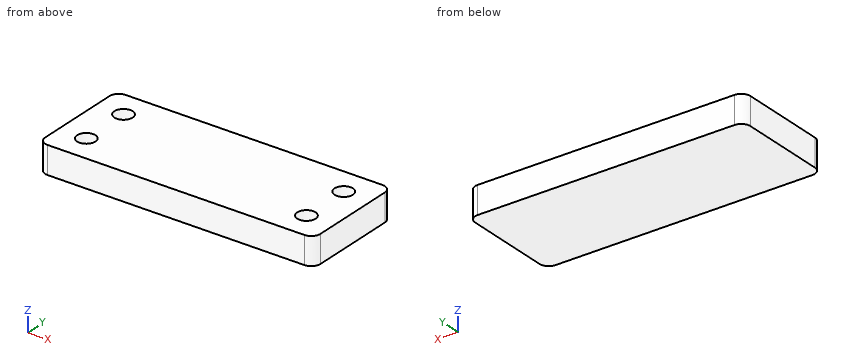
Solid Edge part; units mm, degrees
sketch "Sketch1" plane through (0, 0, 0) normal (0, 0, 1) x (1, 0, 0)
  line L0 (-15, 5.75) -> (15, 5.75)
  line L1 (15, 5.75) -> (15, -5.75)
  line L2 (15, -5.75) -> (-15, -5.75)
  line L3 (-15, -5.75) -> (-15, 5.75)
  dimension "D1" = 15
  dimension "D2" = 15
extrude "Protrusion1" add sketch "Sketch1" along normal blind 3
fillet "Avrundningar_1" radius 1 4 edges at (-15, -5.75, 1.5) (15, -5.75, 1.5) (15, 5.75, 1.5) (-15, 5.75, 1.5)
sketch "Sketch2" plane through (0, 0, 3) normal (0, 0, 1) x (0, 1, 0)
  circle A0 centre (-2.75, 12) radius 1
  circle A1 centre (2.75, 12) radius 1
  circle A2 centre (2.75, -12) radius 1
  circle A3 centre (-2.75, -12) radius 1
  dimension "D1" = 2.75
  dimension "D2" = 2.75
extrude "Utskärning_fäste_fjädrar" cut sketch "Sketch2" against normal blind 1.5
Here's how the part is built. I have some questions about the finished solid (model axes, mm). Round coordinates to 2 decimals unless told otherwise and drop trailing zeros. Order: outer loops, then holes, each group sorted by start corner. A loop starts at its lowest first (then second) coordinate and runs counter-clockwise, first axis right, second up. Notation, with made-up numbers: M -26.5,-35.5 L -22.5,-35.5 A18 cw -22.5,-4.5 Z; hole C 51.5,-33.5 d11. An arc over 180 degrees is marked long. One line per question, with ' | ' between items.
1) Imagine slicing it at B-B, the plane x = -12. Write out the boundary of the cut face in (y, z), plus the area to 3 significant figures.
Checked values:
outline: M -5.75,0 L 5.75,0 L 5.75,3 L 3.75,3 L 3.75,1.5 L 1.75,1.5 L 1.75,3 L -1.75,3 L -1.75,1.5 L -3.75,1.5 L -3.75,3 L -5.75,3 Z | area: 28.5 mm²
2) Imagine slicing it at C-C, the plane y = 2.75. Write out the boundary of the cut face in (x, z), plus the area to 3 significant figures.
Checked values:
outline: M -15,0 L 15,0 L 15,3 L 13,3 L 13,1.5 L 11,1.5 L 11,3 L -11,3 L -11,1.5 L -13,1.5 L -13,3 L -15,3 Z | area: 84.0 mm²
3) I need wall thicknesses on line 1 (Y direction, x = 12, z = 2.6); line 2 (X direction, y = -2.75, z = 1.9); line 3 (X direction, y = 5.25, z = 0.3). Which ranges of each line are inside material? Lowest first, please.
Checked values:
line 1: y = -5.75 to -3.75, -1.75 to 1.75, 3.75 to 5.75 | line 2: x = -15 to -13, -11 to 11, 13 to 15 | line 3: x = -14.87 to 14.87
4) I'm going to push a flat-ended pin straight in: pin 1 Ø0.6 at (x, y) = (12, -2.5) entering from +Z. Where does the tip first touch, or does it pass through?
Checked values:
pin 1: stops at z = 1.5
5) Imagine slicing it at A-A, the plane z = 2.4. Write out the boundary of the cut face in (x, y), plus the area to 3 significant figures.
Checked values:
outline: M -15,-4.75 A1 ccw -14,-5.75 L 14,-5.75 A1 ccw 15,-4.75 L 15,4.75 A1 ccw 14,5.75 L -14,5.75 A1 ccw -15,4.75 Z; hole C -12,-2.75 d2; hole C -12,2.75 d2; hole C 12,-2.75 d2; hole C 12,2.75 d2 | area: 332 mm²
